Design review of the part built by this model. Coordinates are the model's own, in mm. Give positions to 0.01 mm unless a question says otherwise; leave off trailing zeros. Write each loop counter-clockwise with the first axis right and the second up, starting at its lowest first coordinate (ties: lowest second). Pieces come first, ordered by that corner, then holes. Notation, with made-up numbers: (4, -23.5) -> (22, -23.5) arc R10 cw to (22, -9.5) -> close; hole circle Ø3 at (54.5, 47). An arc over 180 degrees is marked (long way). Answer as a JSON object with one key per item and string values.
```python
from build123d import *

# Parameters (mm, degrees)
SKETCH_1_W             = 268
SKETCH_1_H             = 378
EXTRUDE_1_DEPTH        = 246
SKETCH_2_W             = 170
SKETCH_2_H             = 183
CUT_EXTRUDE_1_DEPTH    = 256
EXTRUDE_4_DEPTH        = 6
EXTRUDE_4_DEPTH_BACK   = 3
SKETCH_8_W             = 15.454545454
SKETCH_8_H             = 12
CUT_EXTRUDE_2_DEPTH    = 262
PATTERN_LINEAR_1_COUNT = 5
PATTERN_LINEAR_1_PITCH = 30.909090909


with BuildPart() as part:
    # Эскиз1 → Бобышка-Вытянуть1 (new body)
    with BuildSketch(Plane.XY):
        with Locations((484.747616564, 117.897162102)):
            Rectangle(SKETCH_1_W, SKETCH_1_H)
    extrude(amount=EXTRUDE_1_DEPTH)

    # Эскиз2 → Вырез-Вытянуть1 (cut)
    with BuildSketch(Plane(origin=(618.747616564, 0, 0), x_dir=(0, 0, -1), z_dir=(1, 0, 0))):
        with Locations((-91, 193.997162102)):
            Rectangle(SKETCH_2_W, SKETCH_2_H)
    extrude(amount=-CUT_EXTRUDE_1_DEPTH, mode=Mode.SUBTRACT)

    # Эскиз7 → Бобышка-Вытянуть4 (add, two sides: drawn at the far end of the back side and taken through both)
    with BuildSketch(Plane(origin=(618.747616564, 0, 0), x_dir=(0, 0, -1), z_dir=(1, 0, 0)).offset(-EXTRUDE_4_DEPTH_BACK)):
        Polygon((-240, -71.102837898), (-246, -71.102837898), (-246, 486.497162102), (0, 486.497162102), (0, 306.897162102), (-240, 306.897162102), align=None)
    extrude(amount=EXTRUDE_4_DEPTH + EXTRUDE_4_DEPTH_BACK)

    # Эскиз8 → Вырез-Вытянуть2 (cut)
    with BuildSketch(Plane(origin=(618.747616564, 0, 0), x_dir=(0, 0, -1), z_dir=(1, 0, 0))):
        with Locations((-152.818181818, 96.497162102)):
            Rectangle(SKETCH_8_W, SKETCH_8_H)
    cut_extrude_2 = extrude(amount=-CUT_EXTRUDE_2_DEPTH, mode=Mode.SUBTRACT)

    # Линейный массив1: Вырез-Вытянуть2 ×5
    with Locations(*[(0, 0, -i * PATTERN_LINEAR_1_PITCH) for i in range(1, PATTERN_LINEAR_1_COUNT)]):
        add(cut_extrude_2, mode=Mode.SUBTRACT)


solid = part.part
```
(1) Clearance check with flat-ended pins moving along their axes: pin 1 (6 mm diameter, centred on x = 493, z = 25.5, fed in from +Y); pin 2 (6 mm diameter, centred on x = 553, y = 98.5, fed in from -Z); pin 3 (3.5 mm diameter, centred on y = 93.5, z = 32.5, fed in from +X). State where each tip first meets the part, or that it passes through.
Here are the results:
{"pin 1": "stops at y = 306.9", "pin 2": "stops at z = 0", "pin 3": "stops at x = 356.75"}
(2) We need section A-A, the plane x = 410. State the section outline as (y, z) points.
Here are the results:
{"outline": "(-71.1, 0) -> (306.9, 0) -> (306.9, 246) -> (-71.1, 246) -> close; hole (90.5, 21.45) -> (102.5, 21.45) -> (102.5, 6) -> (285.5, 6) -> (285.5, 176) -> (102.5, 176) -> (102.5, 160.55) -> (90.5, 160.55) -> (90.5, 145.09) -> (102.5, 145.09) -> (102.5, 129.64) -> (90.5, 129.64) -> (90.5, 114.18) -> (102.5, 114.18) -> (102.5, 98.73) -> (90.5, 98.73) -> (90.5, 83.27) -> (102.5, 83.27) -> (102.5, 67.82) -> (90.5, 67.82) -> (90.5, 52.36) -> (102.5, 52.36) -> (102.5, 36.91) -> (90.5, 36.91) -> close"}
(3) We need section B-B, the plane y = 37. State the section outline as (x, z) points.
Here are the results:
{"outline": "(350.75, 0) -> (618.75, 0) -> (618.75, 240) -> (624.75, 240) -> (624.75, 246) -> (350.75, 246) -> close"}
(4) We need section D-D, the plane y = 257. State the section outline as (x, z) points, then the cut area to 3 significant figures.
Here are the results:
{"outline": "(350.75, 0) -> (618.75, 0) -> (618.75, 6) -> (362.75, 6) -> (362.75, 176) -> (618.75, 176) -> (618.75, 240) -> (624.75, 240) -> (624.75, 246) -> (350.75, 246) -> close", "area": "22,400 mm²"}
(5) The part is to be moulded in two halves that separate along Y. For faces 1 (the flat face through (493, 102.497, 45)), 2 (the flat face through (486, 88, 246)), 3 (the flat face through (481, 306.897, 121)), say which applies: +Y half, -Y half, draft (parallel to the pull), parting line (faces both ways), or undercut.
Here are the results:
{"face 1": "undercut", "face 2": "draft", "face 3": "+Y half"}
(6) For line 1 along Z through (x, y) = (576, 222); line 2 along Y through (x, z) = (605, 76.5); line 3 along Y through (x, z) = (489, 29.5), list the stretches that pass through material, from the lowest coordinate up.
Here are the results:
{"line 1": "z = 0 to 6, 176 to 246", "line 2": "y = -71.1 to 102.5, 285.5 to 306.9", "line 3": "y = -71.1 to 90.5, 285.5 to 306.9"}
(7) We need section C-C, the plane z = 216. State the section outline as (x, y) points.
Here are the results:
{"outline": "(350.75, -71.1) -> (618.75, -71.1) -> (618.75, 306.9) -> (624.75, 306.9) -> (624.75, 486.5) -> (615.75, 486.5) -> (615.75, 306.9) -> (350.75, 306.9) -> close"}
